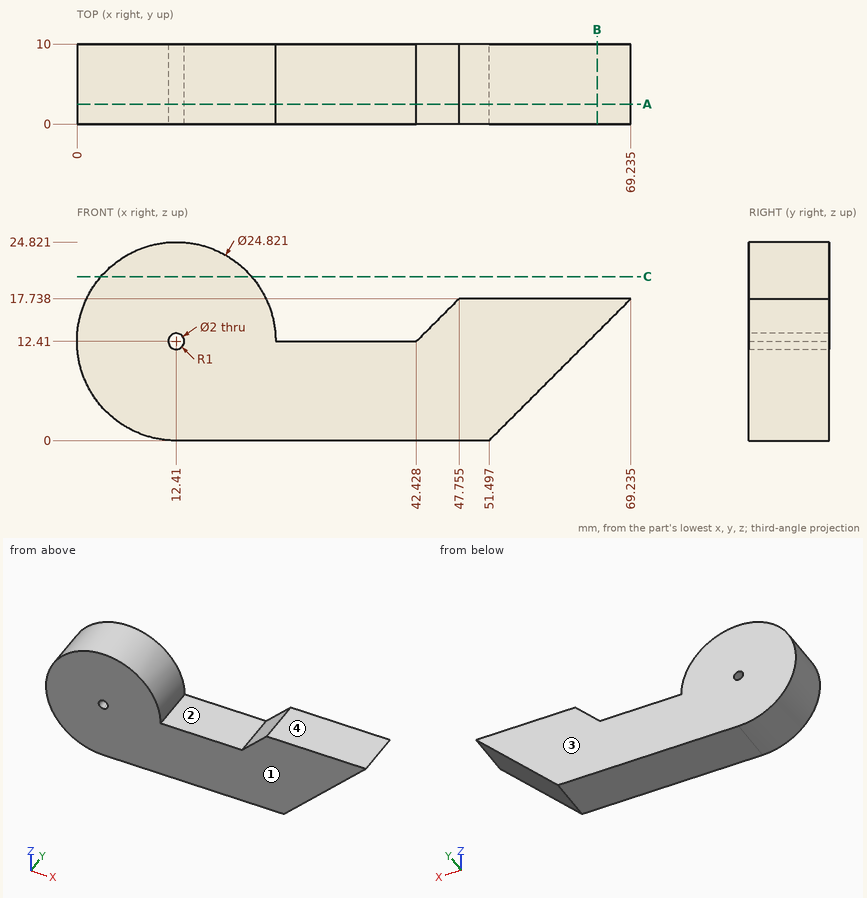
Check sheet for the drawn part. Datum: minimum x, y, z corner. Units: mm. A direction names the side the tool comes from. Round coordinates to 2 decimals unless told otherwise and drop trailing zeros. Order: outer loops, then holes, each group sorted by start corner. A loop starts at its lowest first (then second) coordinate and runs counter-clockwise, first axis right, second up.
(1) Go/stop test with flat-tipped pins: P1, Ø1, axis at x = 42, y = 2.5, coming from the +Z side; P2, Ø6, axis at x = 7.5, y = 7, coming from the -Z side; P3, Ø3, axis at x = 37, y = 3.5, coming from the +Z side. Record where each tip stops, or that it passes through.
(2) Access from +Z, -Z, +X, -X, +Y, -Y to the whole of each face (thin tool, end or side, straight path). Record for the marked faces 3 and 4.
(3) Cross-section at A-A, the plane y = 2.5. Enter the section's corners in (x, z) (1 decimal).
(4) Draft check along X on the marked faces 1 and 2. Enter one of: pulls with the +X half, pulls with the -X half, needs draft (parallel to the pull), parting line crosses it, or undercut.
(5) Cross-section at B-B, the plane x = 65. Enter the section's corners in (y, z).
(6) Cross-section at C-C, the plane z = 20.5. Enter the section's corners in (x, y).
(7) Scan lines: probe 1 along Z at (x, y) = (12.5, 2) (1 decimal); probe 2 along Z at (x, y) = (29, 5.75); probe 3 along Z at (x, y) = (51.5, 3) (1 decimal). Record each from-to range of solid material in increasing order.
Check sheet entries:
1. P1: stops at z = 12.48
1. P2: stops at z = 0.15
1. P3: stops at z = 12.41
2. face 3: +Z, -Z, +X, -X, +Y
2. face 4: +Z, +X, +Y, -Y
3. outline: (12.4, 0) - (51.5, 0) - (69.2, 17.7) - (47.8, 17.7) - (42.4, 12.4) - (24.8, 12.4) arc R12.4 ccw (long way) to start; hole circle Ø2 at (12.4, 12.4)
4. face 1: needs draft
4. face 2: undercut
5. outline: (0, 13.5) - (10, 13.5) - (10, 17.74) - (0, 17.74) - close
6. outline: (3, 0) - (21.82, 0) - (21.82, 10) - (3, 10) - close
7. probe 1: z = 0 to 11.4, 13.4 to 24.8
7. probe 2: z = 0 to 12.41
7. probe 3: z = 0 to 17.7
